Design review of the part built by this model. Coordinates are the model's own, in mm. Face numbers are marked on the shaded views. A direction names the side the tool comes from. Coordinates: 2 decimals unless noted, no trailing zeros. Order: outer loops, then holes, each group sorted by start corner. A loop starts at its lowest first (then second) coordinate and runs counter-clockwise, first axis right, second up. Notation, with made-up numbers: M -26.75,48.5 L -18.75,48.5 A10 cw -18.75,52.5 Z; hole C 11.5,62.25 d10. An arc over 180 degrees is marked long. Answer in a Markdown table with one row per item.
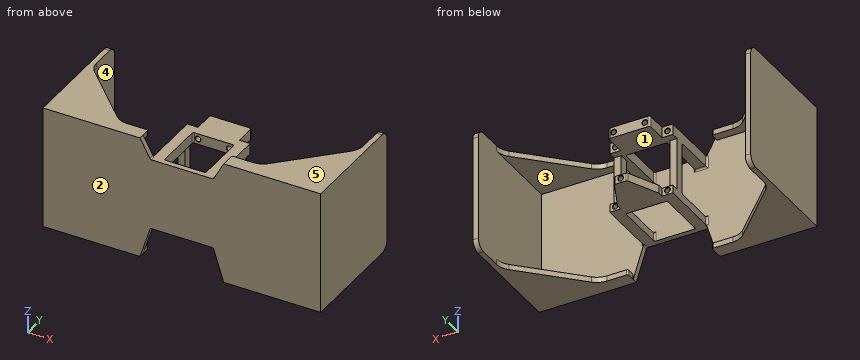
from build123d import *

# Parameters (mm, degrees)
SKETCH1_W           = 154.3
SKETCH1_H           = 68.4
BOSS_EXTRUDE1_DEPTH = 3
SKETCH2_W           = 23
SKETCH2_H           = 4.5
SKETCH2_R           = 1.4
SKETCH2_H_2         = 6
BOSS_EXTRUDE2_DEPTH = 45
BOSS_EXTRUDE3_START = 45
SKETCH2_3_W         = 23
SKETCH2_3_H         = 4.5
SKETCH2_3_R         = 1.4
BOSS_EXTRUDE3_DEPTH = 8.4
BOSS_EXTRUDE4_DEPTH = 29
SKETCH3_W           = 2
SKETCH3_H           = 29.2
CUT_EXTRUDE1_DEPTH  = 29
BOSS_EXTRUDE5_DEPTH = 62
SKETCH4_3_W         = 50.9
SKETCH4_3_H         = 3
BOSS_EXTRUDE6_DEPTH = 5
CUT_EXTRUDE2_DEPTH  = 105.717536736
FILLET1_R           = 5
FILLET2_R           = 1
SKETCH6_W           = 6
SKETCH6_H           = 6
SKETCH6_R           = 1.4
SKETCH6_H_2         = 4.5
BOSS_EXTRUDE7_DEPTH = 4.1
SKETCH8_W           = 29.2
SKETCH8_H           = 24
CUT_EXTRUDE4_DEPTH  = 40
SKETCH9_W           = 23
SKETCH9_H           = 28.1
CUT_EXTRUDE5_DEPTH  = 40
CUT_EXTRUDE6_REACH  = 114.726
FILLET3_R           = 1
CHAMFER1_SIZE       = 0.2
CHAMFER2_SIZE       = 35
FILLET4_R           = 10


with BuildPart() as part:
    # Sketch1 → Boss-Extrude1 (new body)
    with BuildSketch(Plane(origin=(0, 0, 0), x_dir=(1, 0, 0), z_dir=(0, 1, 0))):
        Rectangle(SKETCH1_W, SKETCH1_H)
    extrude(amount=BOSS_EXTRUDE1_DEPTH)

    # Sketch2 → Boss-Extrude2 (add)
    # profile 1 of 2: a face of its own
    with BuildSketch(Plane(origin=(0, 3, 0), x_dir=(1, 0, 0), z_dir=(0, 1, 0))):
        with Locations((0, 13.85)):
            Rectangle(SKETCH2_W, SKETCH2_H)
        with Locations(Location((0, 13.6, 0), (0, 0, 90))):
            Circle(SKETCH2_R, mode=Mode.SUBTRACT)
    # profile 2 of 2: a face of its own
    with BuildSketch(Plane(origin=(0, 3, 0), x_dir=(1, 0, 0), z_dir=(0, 1, 0))):
        with Locations((0, -20.6)):
            Rectangle(SKETCH2_W, SKETCH2_H_2)
        with Locations(Location((8.65, -20.6, 0), (0, 0, 90))):
            Circle(SKETCH2_R, mode=Mode.SUBTRACT)
        with Locations(Location((-8.65, -20.6, 0), (0, 0, 90))):
            Circle(SKETCH2_R, mode=Mode.SUBTRACT)
    extrude(amount=BOSS_EXTRUDE2_DEPTH)

    # Sketch2<3> → Boss-Extrude3 (add)
    with BuildSketch(Plane(origin=(0, 3, 0), x_dir=(1, 0, 0), z_dir=(0, 1, 0)).offset(BOSS_EXTRUDE3_START)):
        with Locations((0, 13.85)):
            Rectangle(SKETCH2_3_W, SKETCH2_3_H)
        with Locations(Location((0, 13.6, 0), (0, 0, 90))):
            Circle(SKETCH2_3_R, mode=Mode.SUBTRACT)
    extrude(amount=BOSS_EXTRUDE3_DEPTH)

    # Sketch2<5> → Boss-Extrude4 (add)
    with BuildSketch(Plane(origin=(0, 3, 0), x_dir=(1, 0, 0), z_dir=(0, 1, 0))):
        Polygon((-11.5, -17.6), (-11.5, 11.6), (-11.5, 16.1), (-17.5, 16.1), (-17.5, -23.6), (-11.5, -23.6), align=None)
        Polygon((11.5, 16.1), (11.5, 11.6), (11.5, -17.6), (11.5, -23.6), (17.5, -23.6), (17.5, 16.1), align=None)
    extrude(amount=BOSS_EXTRUDE4_DEPTH)

    # Sketch3 → Cut-Extrude1 (cut)
    with BuildSketch(Plane(origin=(0, 32, 0), x_dir=(1, 0, 0), z_dir=(0, 1, 0))):
        with Locations((12.5, -3)):
            Rectangle(SKETCH3_W, SKETCH3_H)
        with Locations((-12.5, -3)):
            Rectangle(SKETCH3_W, SKETCH3_H)
    extrude(amount=-CUT_EXTRUDE1_DEPTH, mode=Mode.SUBTRACT)

    # Sketch4 → Boss-Extrude5 (add)
    with BuildSketch(Plane(origin=(0, 3, 0), x_dir=(1, 0, 0), z_dir=(0, 1, 0))):
        Polygon((77.15, -34.2), (77.15, 34.2), (74.15, 34.2), (74.15, 31.2), (74.15, -31.2), (74.15, -34.2), align=None)
        Polygon((-74.15, 31.2), (-74.15, 34.2), (-77.15, 34.2), (-77.15, -34.2), (-74.15, -34.2), (-74.15, -31.2), align=None)
    extrude(amount=BOSS_EXTRUDE5_DEPTH)

    # Sketch4<3> → Boss-Extrude6 (add)
    with BuildSketch(Plane(origin=(0, 3, 0), x_dir=(1, 0, 0), z_dir=(0, 1, 0))):
        with Locations((48.7, 32.7)):
            Rectangle(SKETCH4_3_W, SKETCH4_3_H)
        with Locations((48.7, -32.7)):
            Rectangle(SKETCH4_3_W, SKETCH4_3_H)
        with Locations((-48.7, 32.7)):
            Rectangle(SKETCH4_3_W, SKETCH4_3_H)
        with Locations((-48.7, -32.7)):
            Rectangle(SKETCH4_3_W, SKETCH4_3_H)
    extrude(amount=BOSS_EXTRUDE6_DEPTH)

    # Sketch5 → Cut-Extrude2 (cut, through all)
    with BuildSketch(Plane(origin=(0, 3, 0), x_dir=(1, 0, 0), z_dir=(0, 1, 0))):
        Polygon((23.25, -34.2), (17.5, -23.6), (-17.5, -23.6), (-23.25, -34.2), align=None)
        Polygon((17.5, 16.1), (23.25, 34.2), (-23.25, 34.2), (-17.5, 16.1), align=None)
    extrude(amount=-CUT_EXTRUDE2_DEPTH, mode=Mode.SUBTRACT)

    # Fillet1
    fillet1_edges = [part.edges().sort_by_distance(p)[0] for p in [
        (75.65, 65, -34.2),
        (75.65, 65, 34.2),
        (-75.65, 65, -34.2),
        (-75.65, 65, 34.2),
    ]]
    fillet(fillet1_edges, radius=FILLET1_R)

    # Fillet2
    fillet2_edges = [part.edges().sort_by_distance(p)[0] for p in [
        (23.25, 8, -32.7),
        (23.25, 8, 32.7),
        (-23.25, 8, -32.7),
        (-23.25, 8, 32.7),
        (-17.5, 1.5, 23.6),
        (17.5, 1.5, 23.6),
        (17.5, 1.5, -16.1),
        (-17.5, 1.5, -16.1),
    ]]
    fillet(fillet2_edges, radius=FILLET2_R)

    # Sketch6 → Boss-Extrude7 (add)
    # profile 1 of 4: a face of its own
    with BuildSketch(Plane(origin=(0, 32, 0), x_dir=(1, 0, 0), z_dir=(0, 1, 0))):
        with Locations((-14.5, -20.6)):
            Rectangle(SKETCH6_W, SKETCH6_H)
        with Locations(Location((-14.5, -20.6, 0), (0, 0, 270))):
            Circle(SKETCH6_R, mode=Mode.SUBTRACT)
    # profile 2 of 4: a face of its own
    with BuildSketch(Plane(origin=(0, 32, 0), x_dir=(1, 0, 0), z_dir=(0, 1, 0))):
        with Locations((14.5, -20.6)):
            Rectangle(SKETCH6_W, SKETCH6_H)
        with Locations(Location((14.5, -20.6, 0), (0, 0, 270))):
            Circle(SKETCH6_R, mode=Mode.SUBTRACT)
    # profile 3 of 4: a face of its own
    with BuildSketch(Plane(origin=(0, 32, 0), x_dir=(1, 0, 0), z_dir=(0, 1, 0))):
        with Locations((14.5, 13.85)):
            Rectangle(SKETCH6_W, SKETCH6_H_2)
        with Locations(Location((14.5, 13.6, 0), (0, 0, 270))):
            Circle(SKETCH6_R, mode=Mode.SUBTRACT)
    # profile 4 of 4: a face of its own
    with BuildSketch(Plane(origin=(0, 32, 0), x_dir=(1, 0, 0), z_dir=(0, 1, 0))):
        with Locations((-14.5, 13.85)):
            Rectangle(SKETCH6_W, SKETCH6_H_2)
        with Locations(Location((-14.5, 13.6, 0), (0, 0, 270))):
            Circle(SKETCH6_R, mode=Mode.SUBTRACT)
    extrude(amount=BOSS_EXTRUDE7_DEPTH)

    # Sketch8 → Cut-Extrude4 (cut)
    with BuildSketch(Plane(origin=(17.5, 0, 0), x_dir=(0, 0, -1), z_dir=(1, 0, 0))):
        with Locations((-3, 15)):
            Rectangle(SKETCH8_W, SKETCH8_H)
    extrude(amount=-CUT_EXTRUDE4_DEPTH, mode=Mode.SUBTRACT)

    # Sketch9 → Cut-Extrude5 (cut)
    with BuildSketch(Plane.XY.offset(23.6)):
        with Locations((0, 17.05)):
            Rectangle(SKETCH9_W, SKETCH9_H)
    extrude(amount=-CUT_EXTRUDE5_DEPTH, mode=Mode.SUBTRACT)

    # Sketch10 → Cut-Extrude6 (cut, up to next)
    with BuildSketch(Plane(origin=(0, 0, -16.1), x_dir=(-1, 0, 0), z_dir=(0, 0, -1)), mode=Mode.PRIVATE) as cut_extrude6_sk1:
        Polygon((-11.5, 39.1), (-3.5, 56.4), (-11.5, 56.4), align=None)
    cut_extrude6_tool1 = extrude(cut_extrude6_sk1.sketch, amount=-CUT_EXTRUDE6_REACH, mode=Mode.PRIVATE) & part.part
    # Sketch10 → Cut-Extrude6 (cut, up to next)
    with BuildSketch(Plane(origin=(0, 0, -16.1), x_dir=(-1, 0, 0), z_dir=(0, 0, -1)), mode=Mode.PRIVATE) as cut_extrude6_sk2:
        Polygon((11.5, 56.4), (3.5, 56.4), (11.5, 39.1), align=None)
    cut_extrude6_tool2 = extrude(cut_extrude6_sk2.sketch, amount=-CUT_EXTRUDE6_REACH, mode=Mode.PRIVATE) & part.part
    add(cut_extrude6_tool1.solids().sort_by_distance((8.833333, 50.633333, -16.1))[0], mode=Mode.SUBTRACT)
    add(cut_extrude6_tool2.solids().sort_by_distance((-8.833333, 50.633333, -16.1))[0], mode=Mode.SUBTRACT)

    # Fillet3
    fillet3_edges = [part.edges().sort_by_distance(p)[0] for p in [
        (-14.5, 3, -11.6),
        (-11.5, 48, 20.6),
        (11.5, 48, 20.6),
        (-14.5, 3, 17.6),
        (17.5, 3, 20.6),
        (-17.5, 3, 20.6),
        (-15.5, 27, 17.6),
        (15.5, 27, 17.6),
        (-15.5, 27, -11.6),
        (15.5, 27, -11.6),
        (14.5, 3, 17.6),
        (14.5, 3, -11.6),
        (-11.5, 3, -13.85),
        (11.5, 31.1, -13.85),
        (-11.5, 31.1, -13.85),
        (11.5, 3, -13.85),
        (-11.5, 3, 20.6),
        (-11.5, 31.1, 20.6),
        (11.5, 31.1, 20.6),
        (11.5, 3, 20.6),
        (3.5, 56.4, -13.85),
        (11.5, 39.1, -13.85),
        (-11.5, 39.1, -13.85),
        (-3.5, 56.4, -13.85),
        (-17.5, 3, -13.85),
        (17.5, 3, -13.85),
    ]]
    fillet(fillet3_edges, radius=FILLET3_R)

    # Chamfer1
    chamfer1_edges = [part.edges().sort_by_distance(p)[0] for p in [
        (-8.65, 48, 22),
        (8.65, 48, 22),
        (-14.5, 32, 19.2),
        (-14.5, 36.1, 19.2),
        (14.5, 32, 19.2),
        (14.5, 36.1, 19.2),
        (-14.5, 32, -15),
        (-14.5, 36.1, -15),
        (14.5, 32, -15),
        (14.5, 36.1, -15),
        (-8.65, 31.1, 22),
        (8.65, 31.1, 22),
        (0, 31.1, -12.2),
        (0, 56.4, -12.2),
    ]]
    chamfer(chamfer1_edges, length=CHAMFER1_SIZE)

    # Chamfer2
    chamfer2_edges = [part.edges().sort_by_distance(p)[0] for p in [
        (74.15, 8, -32.7),
        (74.15, 8, 32.7),
        (-74.15, 8, -32.7),
        (-74.15, 8, 32.7),
    ]]
    chamfer(chamfer2_edges, length=CHAMFER2_SIZE)

    # Fillet4
    fillet4_edges = [part.edges().sort_by_distance(p)[0] for p in [
        (74.15, 43, 32.7),
        (74.15, 43, -32.7),
        (39.15, 8, -32.7),
        (39.15, 8, 32.7),
        (-39.15, 8, -32.7),
        (-74.15, 43, 32.7),
        (-74.15, 43, -32.7),
        (-39.15, 8, 32.7),
    ]]
    fillet(fillet4_edges, radius=FILLET4_R)


solid = part.part
(1) Insertion check: pin 1 Ø6 at (x, z) = (-52.5, -23.5) entering from +Y; pin 2 Ø3 at (x, y) = (40.5, 14) entering from +Z; pin 3 Ø18.5 at (x, y) = (3.5, 24) entering from -Z; pin 4 Ø5 at (x, z) = (-3, 21.5) entering from +Y. Each pin has a flat end and moves straight along its axis. Give the tip position at first contact, or say it passes through.
Return value:
| item | result |
|---|---|
| pin 1 | stops at y = 3 |
| pin 2 | passes through |
| pin 3 | stops at z = -16.1 |
| pin 4 | stops at y = 48 |
(2) For the marked faces 4 and 5, list the 3-axis set-ups (+Z, -Z, +X, -X, +Y, -Y) from which the entire face can be reached by the end or side of a thin tool; tool diameter is ignored.
Return value:
| item | result |
|---|---|
| face 4 | +Y |
| face 5 | +Z, +X, -X, +Y, -Y |
(3) Add section C-C, the plane z = -19. Give the boundary of the cut face in (x, y), and give its area (3 significant figures).
Return value:
| item | result |
|---|---|
| outline | M -77.15,0 L -18.42,0 L -18.42,3 L -74.15,3 L -74.15,65 L -77.15,65 Z; M 18.42,0 L 77.15,0 L 77.15,65 L 74.15,65 L 74.15,3 L 18.42,3 Z |
| area | 724 mm2 |
(4) Add section D-D, the plane y = 43.5. Give the boundary of the cut face in (x, z).
Return value:
| item | result |
|---|---|
| outline | M -77.15,-34.2 L -73.46,-34.2 L -73.46,-31.2 L -74.15,-31.2 L -74.15,31.2 L -73.46,31.2 L -73.46,34.2 L -77.15,34.2 Z; M -11.5,17.6 L 11.5,17.6 L 11.5,23.6 L -11.5,23.6 Z; M -9.47,-16.1 L 9.47,-16.1 L 9.47,-11.6 L -9.47,-11.6 Z; M 73.46,-34.2 L 77.15,-34.2 L 77.15,34.2 L 73.46,34.2 L 73.46,31.2 L 74.15,31.2 L 74.15,-31.2 L 73.46,-31.2 Z; hole C -8.65,20.6 d2.8; hole C 0,-13.6 d2.8; hole C 8.65,20.6 d2.8 |
(5) Draft analysis for pull direction Y (two halves, no side actions). For the marked faces 1, 2 and 3, state which applies: pulls with the +Y half, pulls with the -Y half, needs draft (parallel to the pull), parting line crosses it, or undercut.
Return value:
| item | result |
|---|---|
| face 1 | undercut |
| face 2 | pulls with the -Y half |
| face 3 | needs draft |
(6) Add section A-A, the plane y = 23.5. Give the number of separate pieces and of enclosed holes in the cut face, and give its area (3 significant figures).
Return value:
| item | result |
|---|---|
| separate pieces | 6 |
| enclosed holes | 0 |
| area | 770 mm2 |
(7) For line 1 along Z through (x, y) = (-8.65, 36.25); line 2 along X through (y, z) = (34.65, -13.6); line 3 along X through (y, z) = (52, -12), list the stretches that pass through material, from the lowest coordinate up. Write a range as from..to.
Return value:
| item | result |
|---|---|
| line 1 | z = -16.1..-11.6, 17.6..19.2, 22..23.6 |
| line 2 | x = -77.15..-74.15, -17.5..-15.9, -13.1..-1.4, 1.4..13.1, 15.9..17.5, 74.15..77.15 |
| line 3 | x = -77.15..-74.15, -5.53..5.53, 74.15..77.15 |
(8) Add section B-B, the plane x = -47. Give the boundary of the cut face in (y, z), and give its area (3 significant figures).
Return value:
| item | result |
|---|---|
| outline | M 0,-34.2 L 15.85,-34.2 L 15.85,-31.2 L 3,-31.2 L 3,31.2 L 15.85,31.2 L 15.85,34.2 L 0,34.2 Z |
| area | 282 mm2 |
